Model file for the job. Use its own axes, mm. A direction names the side the tool comes from. Coordinates: 2 decimals unless noted, no trailing zeros. Write each loop counter-clockwise with the first axis right and the second up, starting at its lowest first coordinate (ties: lowest second). Pieces come first, ordered by that corner, then holes. Notation, with made-up numbers: M 35,-8 L 77,-8 A5 cw 77,1 Z; hole C 58.5,16 d2. An arc over 180 degrees is marked long. Put each result on its own line as item: value. Start each with the question number.
Q1. Cut at B-B (y = 0). Give the number of separate pieces and of enclosed holes in the cut face, then the cut area to 3 significant figures.
Q2. Drill centre lines: line 1 along Z through (x, y) = (-15, 0); line 2 along X through (y, z) = (6.25, 27); line 3 along Y through (x, z) = (-16, 44). Where is each one in solid material? Low to high.
Q3. Pull direction X, two halves, no side cores. Call faces 5 (the flat face through (-9.4, -0.1, 8.7)), 6 (the cylindrical face through (16.32, -0.298, 46.317)), 7 (the flat face through (0, 0, 5)), 8 (the flat face through (-23.15, -0.14, 8.6)): pulls with the +X half, pulls with the -X half, needs draft (parallel to the pull), parting line crosses it, or undercut.
Q4. Cut at C-C (z = 44.05). Write the cut outline in (x, y), then the cut area to 3 significant figures.
Q5. Which spindle directions (+Z, -Z, +X, -X, +Y, -Y) get a long thin tool onto all of the face, cutting with end or side? Do faces 1 (the flat face through (21.25, 0, 32)), 2 (the flat face through (-11.5, -10, 19.2)), 3 (the flat face through (9.35, -0.14, 8.6)), 4 (the flat face through (-21.25, 0, 31)). Say none if no direction does.
Q6. Cut at A-A (z = 29). Write the cut outline in (x, y).
Q7. Cut at D-D (x = -14.5). Write the cut outline in (y, z).
Q8. Drop flat-ended pins along their axis: pin 1 (5.5 mm diameter, centred on y = 0, z = 44.05, fed in from +X); pin 2 (4.5 mm diameter, centred on x = -1.5, y = -1, fed in from +Z); pin 3 (10 mm diameter, centred on y = 1.5, z = 32, fed in from -X); pin 4 (4 mm diameter, centred on x = -8.5, z = 37, fed in from -Y). Give the stop position or say it passes through.
```python
from build123d import *

# Parameters (mm, degrees)
F0_W      = 50
F0_H      = 20
F1_DEPTH  = 5
F2_W      = 17.5
F2_H      = 20
F3_DEPTH  = 20
F3_FACE_W = 17.5
F3_FACE_H = 20
F4_DEPTH  = 25.4
F5_R      = 2.286
F6_DEPTH  = 50.001
F8_DEPTH  = 20.001


with BuildPart() as f1:
    # F0 (on Top) → F1 (new body)
    with BuildSketch(Plane.XY):
        Rectangle(F0_W, F0_H)
    extrude(amount=F1_DEPTH)

    # F2 (on face) → F3 (join)
    with BuildSketch(Plane.XY.offset(5)):
        with Locations((16.25, 0)):
            Rectangle(F2_W, F2_H)
        with Locations((-16.25, 0)):
            Rectangle(F2_W, F2_H)
    extrude(amount=F3_DEPTH)

    # F3_face (on face) → F4 (join)
    with BuildSketch(Plane(origin=(16.25, 0, 25), x_dir=(1, 0, 0), z_dir=(0, 0, 1))):
        Rectangle(F3_FACE_W, F3_FACE_H)
        with Locations((-32.5, 0)):
            Rectangle(F3_FACE_W, F3_FACE_H)
    extrude(amount=F4_DEPTH)

    # F5 (on face) → F6 (cut, through all)
    with BuildSketch(Plane.YZ.offset(25)):
        with Locations((0, 44.05)):
            Circle(F5_R)
        with Locations((0, 18.65)):
            Circle(F5_R)
    extrude(amount=-F6_DEPTH, mode=Mode.SUBTRACT)

    # F7 (on face) → F8 (cut, through all)
    with BuildSketch(Plane.XZ.offset(10)):
        Polygon((-25, 50.4), (-25, 5), (-21.25, 12.3), (-21.25, 50.4), align=None)
        Polygon((-11.25, 12.3), (-7.5, 5), (-7.5, 50.4), (-11.25, 50.4), align=None)
        Polygon((7.5, 50.4), (7.5, 5), (11.25, 12.3), (11.25, 50.4), align=None)
        Polygon((21.25, 12.3), (25, 5), (25, 50.4), (21.25, 50.4), align=None)
    extrude(amount=-F8_DEPTH, mode=Mode.SUBTRACT)


solid = f1.part
```
Computed values:
1. separate pieces: 5
1. enclosed holes: 0
1. area: 1,030 mm2
2. line 1: 0 to 16.36, 20.94 to 41.76, 46.34 to 50.4
2. line 2: -21.25 to -11.25, 11.25 to 21.25
2. line 3: -10 to -2.29, 2.29 to 10
3. face 5: undercut
3. face 6: needs draft
3. face 7: undercut
3. face 8: pulls with the -X half
4. outline: M -21.25,-10 L -11.25,-10 L -11.25,-2.29 L -21.25,-2.29 Z; M -21.25,2.29 L -11.25,2.29 L -11.25,10 L -21.25,10 Z; M 11.25,-10 L 21.25,-10 L 21.25,-2.29 L 11.25,-2.29 Z; M 11.25,2.29 L 21.25,2.29 L 21.25,10 L 11.25,10 Z
4. area: 309 mm2
5. face 1: +Z, +X, +Y, -Y
5. face 2: +Z, -Z, +X, -X, -Y
5. face 3: +Z, +Y, -Y
5. face 4: +Z, -X, +Y, -Y
6. outline: M -21.25,-10 L -11.25,-10 L -11.25,10 L -21.25,10 Z; M 11.25,-10 L 21.25,-10 L 21.25,10 L 11.25,10 Z
7. outline: M -10,0 L 10,0 L 10,50.4 L -10,50.4 Z; hole C 0,18.65 d4.57; hole C 0,44.05 d4.57
8. pin 1: x = 21.25
8. pin 2: z = 5
8. pin 3: x = -21.25
8. pin 4: through
